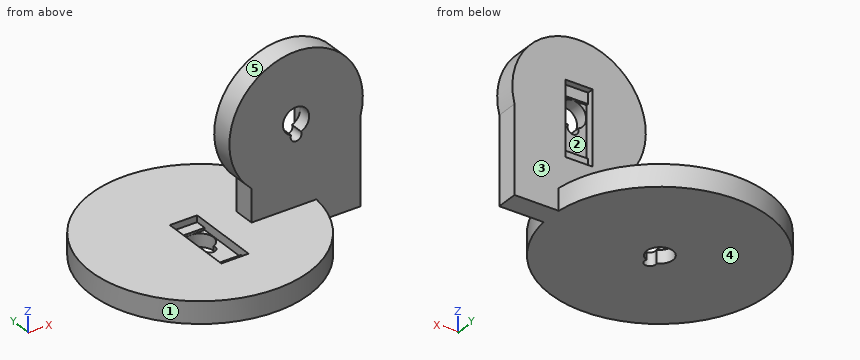
Autodesk Fusion 360 part; units mm, degrees
sketch "Sketch1" plane through (0, 0, 0) normal (0, 0, 1) x (1, 0, 0)
  circle A0 centre (0, 0) radius 50
  dimension "d1" = 100
extrude "Extrude1" add sketch "Sketch1" along normal blind 10
sketch "Sketch2" plane through (0, 0, 10) normal (0, 0, 1) x (-1, 0, 0)
  circle A0 centre (0, 0) radius 50
  line L0 (-6.25, -11) -> (6.25, -11)
  line L1 (6.25, -11) -> (6.25, 23)
  line L2 (6.25, 23) -> (-6.25, 23)
  line L3 (-6.25, 23) -> (-6.25, -11)
  line L4 (-6.25, -11) -> (6.25, 23) construction
  line L5 (6.25, -11) -> (-6.25, 23) construction
  line L6 (6.25, -6) -> (-6.25, -6)
  line L7 (6.25, 18) -> (-6.25, 18)
  point P0 (0, 6)
  point P1 (0, 6)
  dimension "d4" = 6
  dimension "d5" = 12.5
  dimension "d6" = 34
  dimension "d7" = 5
  dimension "d8" = 5
extrude "Extrude2" cut sketch "Sketch2" against normal blind 3 contours L0 L1 L3 L6 | L1 L3 L6 L7 | L1 L2 L3 L7
sketch "Sketch3" plane through (0, 0, 7) normal (0, 0, 1) x (-1, 0, 0)
  line L0 (-6.25, 23) -> (-6.25, -11)
  line L1 (-6.25, -11) -> (6.25, -11)
  line L2 (6.25, -11) -> (6.25, 23)
  line L3 (6.25, 23) -> (-6.25, 23)
  line L4 (6.25, -6) -> (-6.25, -6)
  line L5 (6.25, 18) -> (-6.25, 18)
  dimension "d11" = 5
  dimension "d12" = 5
extrude "Extrude3" cut sketch "Sketch3" against normal blind 1 contours L0 L2 L4 L5
sketch "Sketch4" plane through (0, 0, 6) normal (0, 0, 1) x (-1, 0, 0)
  line L0 (6.25, -6) -> (6.25, 18)
  line L1 (6.25, 18) -> (-6.25, 18)
  line L2 (-6.25, 18) -> (-6.25, -6)
  line L3 (-6.25, -6) -> (6.25, -6)
  circle A0 centre (0, 0) radius 6
  circle A1 centre (0, 6.5) radius 2.5
  dimension "d15" = 12
  dimension "d16" = 5
  dimension "d17" = 6.5
extrude "Extrude4" cut sketch "Sketch4" against normal blind 6 contours A0 A1 | A0 A1 | A0 A1
sketch "Sketch5" plane through (0, 0, 7) normal (0, 0, 1) x (-1, 0, 0)
  line L0 (-6.25, 18) -> (6.25, 18)
  line L1 (6.25, 18) -> (6.25, 23)
  line L2 (6.25, 23) -> (-6.25, 23)
  line L3 (-6.25, 23) -> (-6.25, 18)
  circle A0 centre (0, 20.5) radius 1.25
  dimension "d20" = 2.5
  dimension "d21" = 2.5
sketch "Sketch6" plane through (0, 0, 7) normal (0, 0, 1) x (-1, 0, 0)
  line L0 (6.25, -6) -> (-6.25, -6)
  line L1 (-6.25, -6) -> (-6.25, -11)
  line L2 (-6.25, -11) -> (6.25, -11)
  line L3 (6.25, -11) -> (6.25, -6)
  circle A0 centre (0, -8.5) radius 1.25
  dimension "d22" = 2.5
  dimension "d23" = 2.5
extrude "Extrude5" cut sketch "Sketch6" along normal through all contours A0
extrude "Extrude6" cut sketch "Sketch5" along normal through all contours A0
thread "Thread1" thread offset 0 thread length 10
thread "Thread2" thread offset 0 thread length 10
sketch "Sketch7" plane through (0, 0, 0) normal (0, 1, 0) x (1, 0, 0)
  line L0 (20, 0) -> (70, 0)
  line L1 (70, 0) -> (70, -40)
  arc A0 (20, -25) -> (70, -40) centre (40.4442, -47.6861) ccw
  line L2 (20, -25) -> (20, 0)
  dimension "d30" = 50
  dimension "d31" = 40
  dimension "d32" = 20
extrude "Extrude7" add sketch "Sketch7" along normal mid plane 10
sketch "Sketch8" plane through (0, 5, 0) normal (0, 1, 0) x (-1, 0, 0)
  line L0 (-49.7494, 10) -> (-20, 10)
  line L1 (-20, 10) -> (-20, 25)
  arc A0 (-20, 25) -> (-70, 40) centre (-40.4442, 47.6861) ccw
  line L2 (-70, 40) -> (-70, 0)
  line L3 (-70, 0) -> (-49.7494, 0)
  line L4 (-49.7494, 0) -> (-49.7494, 10)
  line L5 (-34.1942, 24.6861) -> (-46.6942, 24.6861)
  line L6 (-46.6942, 24.6861) -> (-46.6942, 58.6861)
  line L7 (-46.6942, 58.6861) -> (-34.1942, 58.6861)
  line L8 (-34.1942, 58.6861) -> (-34.1942, 24.6861)
  line L9 (-34.1942, 24.6861) -> (-46.6942, 58.6861) construction
  line L10 (-46.6942, 24.6861) -> (-34.1942, 58.6861) construction
  point P0 (-40.4442, 47.6861)
  point P1 (-40.4442, 41.6861)
  point P2 (-40.4442, 41.6861)
  dimension "d35" = 6
  dimension "d36" = 12.5
  dimension "d37" = 34
extrude "Extrude8" cut sketch "Sketch8" against normal blind 3 contours L5 L6 L7 L8
sketch "Sketch9" plane through (0, 2, 0) normal (0, 1, 0) x (-1, 0, 0)
  line L0 (-34.1942, 58.6861) -> (-46.6942, 58.6861)
  line L1 (-46.6942, 58.6861) -> (-46.6942, 24.6861)
  line L2 (-46.6942, 24.6861) -> (-34.1942, 24.6861)
  line L3 (-34.1942, 24.6861) -> (-34.1942, 58.6861)
  line L4 (-46.6942, 53.6861) -> (-34.1942, 53.6861)
  line L5 (-46.6942, 29.6861) -> (-34.1942, 29.6861)
  dimension "d40" = 5
  dimension "d41" = 5
extrude "Extrude9" cut sketch "Sketch9" against normal blind 1 contours L1 L3 L4 L5
sketch "Sketch10" plane through (0, 1, 0) normal (0, 1, 0) x (-1, 0, 0)
  line L0 (-46.6942, 53.6861) -> (-46.6942, 29.6861)
  line L1 (-46.6942, 29.6861) -> (-34.1942, 29.6861)
  line L2 (-34.1942, 29.6861) -> (-34.1942, 53.6861)
  line L3 (-34.1942, 53.6861) -> (-46.6942, 53.6861)
  circle A0 centre (-40.4442, 47.6861) radius 6
  circle A1 centre (-40.4442, 41.1861) radius 2.5
  dimension "d44" = 12
  dimension "d45" = 5
  dimension "d46" = 6.5
extrude "Extrude10" cut sketch "Sketch10" against normal blind 6 contours A0 A1 | A0 A1 | A0 A1
sketch "Sketch11" plane through (0, 2, 0) normal (0, 1, 0) x (-1, 0, 0)
  line L0 (-34.1942, 29.6861) -> (-46.6942, 29.6861)
  line L1 (-46.6942, 29.6861) -> (-46.6942, 24.6861)
  line L2 (-46.6942, 24.6861) -> (-34.1942, 24.6861)
  line L3 (-34.1942, 24.6861) -> (-34.1942, 29.6861)
  circle A0 centre (-40.4442, 27.1861) radius 1.25
  dimension "d49" = 2.5
  dimension "d50" = 2.5
sketch "Sketch12" plane through (0, 2, 0) normal (0, 1, 0) x (-1, 0, 0)
  line L0 (-46.6942, 53.6861) -> (-34.1942, 53.6861)
  line L1 (-34.1942, 53.6861) -> (-34.1942, 58.6861)
  line L2 (-34.1942, 58.6861) -> (-46.6942, 58.6861)
  line L3 (-46.6942, 58.6861) -> (-46.6942, 53.6861)
  circle A0 centre (-40.4442, 56.1861) radius 1.25
  dimension "d51" = 2.5
  dimension "d52" = 2.5
extrude "Extrude11" cut sketch "Sketch12" along normal through all contours A0
extrude "Extrude12" cut sketch "Sketch11" along normal through all contours A0
thread "Thread3" thread offset 0 thread length 10
sketch "Sketch13" plane through (0, 5, 0) normal (0, 1, 0) x (-1, 0, 0)
  line L0 (-46.6942, 24.6861) -> (-46.6942, 58.6861)
  line L1 (-46.6942, 58.6861) -> (-34.1942, 58.6861)
  line L2 (-34.1942, 58.6861) -> (-34.1942, 24.6861)
  line L3 (-34.1942, 24.6861) -> (-46.6942, 24.6861)
  line L4 (-49.7494, 10) -> (-20, 10)
  line L5 (-20, 10) -> (-20, 25)
  arc A0 (-20, 25) -> (-70, 40) centre (-40.4442, 47.6861) ccw
  line L6 (-70, 40) -> (-70, 0)
  line L7 (-70, 0) -> (-49.7494, 0)
  line L8 (-49.7494, 0) -> (-49.7494, 10)
CAD build for the part. Positions are in the model's coordinates, mm. Face numbers are marked on the shaded views. A direction names the side the tool comes from. Round coordinates to 2 decimals unless told otherwise and drop trailing zeros. Order: outer loops, then holes, each group sorted by start corner. A loop starts at its lowest first (then second) coordinate and runs counter-clockwise, first axis right, second up.
Q1. Slice it at B-B (z = 18.5). Write the cut outline in (x, y), and give its area (3 significant figures).
Q2. Wall check: L1, parallel to X at y = 0, z = 1.45; L2, parallel to Y at x = 0, z = 3; L3, parallel to Y at x = 51.5, z = 29.5. Give the ranges that are in metal, low to high.
Q3. Slice it at D-D (y = 15). Write the cut outline in (x, z), and give its area (3 significant figures).
Q4. Drop flat-ended pins along their axis: pin 1 (1.5 mm diameter, centred on x = 43, y = 3, fed in from +Z); pin 2 (4 mm diameter, centred on x = 39.5, z = 38, fed in from +Y); pin 3 (0.9 mm diameter, centred on x = 1.5, z = 8, fed in from -Y). Give the stop position or say it passes through.
Q5. Which spindle directions (+Z, -Z, +X, -X, +Y, -Y) get a long thin tool onto all of the face, cutting with end or side? Do the marked faces 1 and 2. Say none if no direction does.
Q6. Slice it at A-A (x = 14.5). Write the cut outline in (y, z).
Q7. Two-plate mould, pull along Z, no slides. Class the marked faces 3, 4 and 5: pulls with the +Z half, pulls with the -Z half, needs draft (parallel to the pull), parting line crosses it, or undercut.
Q8. Slice it at C-C (y = -16). Write the cut outline in (x, z).
Results below:
1. outline: (20, -5) - (70, -5) - (70, 5) - (20, 5) - close
1. area: 500 mm2
2. L1: x = -50 to -6, 6 to 70
2. L2: y = -50 to -9, 6 to 50
2. L3: y = -5 to 5
3. outline: (-47.7, 0) - (47.7, 0) - (47.7, 10) - (-47.7, 10) - close
3. area: 954 mm2
4. pin 1: stops at z = 78.17
4. pin 2: stops at y = 1
4. pin 3: stops at y = -49.99
5. face 1: +Z, -Z
5. face 2: +Y
6. outline: (-47.85, 0) - (47.85, 0) - (47.85, 10) - (-47.85, 10) - close; (-5, 31.58) - (5, 31.58) - (5, 63.8) - (-5, 63.8) - close
7. face 3: needs draft
7. face 4: pulls with the -Z half
7. face 5: undercut
8. outline: (-47.37, 0) - (47.37, 0) - (47.37, 10) - (6.25, 10) - (6.25, 6) - (-6.25, 6) - (-6.25, 10) - (-47.37, 10) - close
